from build123d import *

# Parameters (mm, degrees)
F0_W      = 120
F0_H      = 70
F1_DEPTH  = 2
F3_DEPTH  = 1
F5_DEPTH  = 2
F6_W      = 20
F6_H      = 1
F7_DEPTH  = 3
F9_DEPTH  = 5
F11_DEPTH = 5
F12_R     = 1.5
F13_DEPTH = 5.001


# Not quite as in the source:
# - a feature names something its author has since deleted; it is built from what else it names


with BuildPart() as f1:
    # F0 (on Front) → F1 (new body)
    with BuildSketch(Plane.XZ):
        Rectangle(F0_W, F0_H)
    extrude(amount=F1_DEPTH)

    # F2 (on face) → F3 (join)
    with BuildSketch(Plane.XZ.offset(2)):
        Polygon((-59, -34), (-59, 35), (-60, 35), (-60, -35), (60, -35), (60, 35), (59, 35), (59, -34), align=None)
    extrude(amount=F3_DEPTH)

    # F4 (on face) → F5 (join)
    with BuildSketch(Plane.XZ.offset(3)):
        Polygon((-57, 35), (-60, 35), (-60, -35), (60, -35), (60, 35), (57, 35), (57, -32), (-57, -32), align=None)
    extrude(amount=F5_DEPTH)

    # F6 (on face) → F7 (join)
    with BuildSketch(Plane.XZ.offset(2)):
        with Locations((0, 34.5)):
            Rectangle(F6_W, F6_H)
    extrude(amount=F7_DEPTH)

    # F8 (on face) → F9 (join)
    with BuildSketch(Plane.XZ.offset(5)):
        with BuildLine():
            ThreePointArc((0, 45), (-7.0710678119, 42.0710678119), (-10, 35))
            Line((-10, 35), (10, 35))
            ThreePointArc((10, 35), (7.0710678119, 42.0710678119), (0, 45))
        make_face()
    extrude(amount=-F9_DEPTH)

    # F10 (on face) → F11 (join)
    with BuildSketch(Plane.XZ.offset(5)):
        with BuildLine():
            Line((10, -35), (-10, -35))
            ThreePointArc((-10, -35), (-7.0710678119, -42.0710678119), (0, -45))
            ThreePointArc((0, -45), (7.0710678119, -42.0710678119), (10, -35))
        make_face()
    extrude(amount=-F11_DEPTH)

    # F12 (on face) → F13 (cut, through all)
    with BuildSketch(Plane.XZ.offset(5)):
        with Locations((-4, -39)):
            Circle(F12_R)
        with Locations((4, -39)):
            Circle(F12_R)
        with Locations((-4, 39)):
            Circle(F12_R)
        with Locations((4, 39)):
            Circle(F12_R)
    extrude(amount=-F13_DEPTH, mode=Mode.SUBTRACT)


solid = f1.part
Work out the finished part from the listing and answer in its coordinate system (mm). A direction names the side the tool comes from. Round coordinates to 2 decimals unless told otherwise and drop trailing zeros. Write each loop counter-clockwise with the first axis right and the second up, starting at its lowest first coordinate (ties: lowest second). Pieces come first, ordered by that corner, then holes.
1) Straight lines are drawn through the part: line 1 (X direction, y = -3.45, z = -26.5); line 2 (Z direction, x = 4, y = -1.85); line 3 (Z direction, x = -35, y = -1.3). For each, find the intervals that lie inside material, in ascending order.
2) A cutting plane is placed at B-B (x = -4). Give the vertices of the cut face in (y, z), plus the area to 3 significant figures.
3) Given pin 1 Ø2 at (x, y) = (-28.5, -4) entering from +Z; pin 2 Ø6 at (x, z) = (-37.5, -27) entering from -Y; pin 3 Ø2 at (x, y) = (-1.5, -3.5) entering from -Z, each flat-ended and moving along its own axis, determine where each tip first touches the part or whether it passes through.
4) A cutting plane is placed at D-D (z = -16). Give the vertices of the cut face in (x, y), plus the area to 3 significant figures.
5) A cutting plane is placed at C-C (z = -39). Give the vertices of the cut face in (x, y), plus the area to 3 significant figures.
6) The mould has two halves that part along X. Classify faces 4 (the cylindrical face through (-4.325, -2.535, -40.464)), 5 (the flat face through (-35, -1, 35)), 6 (the flat face through (60, -2, 0)): pulls with the +X half, pulls with the -X half, needs draft (parallel to the pull), parting line crosses it, or undercut.
7) A tool of negligible diameter and unlimited length cuts with its end or side. For faces 1 (the flat face through (0, -3, 34)), 2 (the flat face through (35, -2, -35)), 3 (the flat face through (-35, -2, -35)), from which of +Z, -Z, +X, -X, +Y, -Y can it reach the whole face along a straight path? Write none if from no direction.
8) A cutting plane is placed at A-A (y = -3.85). Give the vertices of the cut face in (x, z), plus the area to 3 significant figures.
Completed:
1. line 1: x = -60 to -57, 57 to 60
1. line 2: z = -44.17 to -40.5, -37.5 to 37.5, 40.5 to 44.17
1. line 3: z = -35 to 35
2. outline: (-5, -44.17) - (0, -44.17) - (0, -40.5) - (-5, -40.5) - close; (-5, -37.5) - (0, -37.5) - (0, 37.5) - (-5, 37.5) - (-5, 34) - (-2, 34) - (-2, -34) - (-3, -34) - (-3, -32) - (-5, -32) - close; (-5, 40.5) - (0, 40.5) - (0, 44.17) - (-5, 44.17) - close
2. area: 212 mm2
3. pin 1: stops at z = -32
3. pin 2: stops at y = -2
3. pin 3: stops at z = -44.99
4. outline: (-60, -5) - (-57, -5) - (-57, -3) - (-59, -3) - (-59, -2) - (59, -2) - (59, -3) - (57, -3) - (57, -5) - (60, -5) - (60, 0) - (-60, 0) - close
4. area: 254 mm2
5. outline: (-9.17, -5) - (-5.5, -5) - (-5.5, 0) - (-9.17, 0) - close; (-2.5, -5) - (2.5, -5) - (2.5, 0) - (-2.5, 0) - close; (5.5, -5) - (9.17, -5) - (9.17, 0) - (5.5, 0) - close
5. area: 61.7 mm2
6. face 4: undercut
6. face 5: needs draft
6. face 6: pulls with the +X half
7. face 1: -Y
7. face 2: -Z, +X, +Y, -Y
7. face 3: -Z, -X, +Y, -Y
8. outline: (-60, -35) - (-10, -35) arc R10 ccw to (10, -35) - (60, -35) - (60, 35) - (57, 35) - (57, -32) - (-57, -32) - (-57, 35) - (-60, 35) - close; (-10, 34) - (10, 34) - (10, 35) arc R10 ccw to (-10, 35) - close; hole circle Ø3 at (-4, -39); hole circle Ø3 at (-4, 39); hole circle Ø3 at (4, -39); hole circle Ø3 at (4, 39)
8. area: 1,070 mm2
